Check sheet for the modelled part. Datum: model origin and axes. Units: mm. A direction names the side the tool comes from. Round coordinates to 2 decimals unless told otherwise and drop trailing zeros. Order: outer loops, then holes, each group sorted by start corner. A loop starts at its lowest first (then second) coordinate and runs counter-clockwise, first axis right, second up. Notation, with made-up numbers: (58.5, 9) -> (99.5, 9) arc R24 cw to (99.5, 21) -> close; hole circle Ø1 at (68, 45.5). An arc over 180 degrees is marked (long way). Answer in a Markdown table with one row per item.
Autodesk Fusion 360 part; units mm, degrees
sketch "Sketch1" plane through (0, 0, 0) normal (0, 1, 0) x (1, 0, 0)
  line L0 (17.5, -87.5) -> (-17.5, -87.5)
  line L1 (-17.5, 87.5) -> (17.5, 87.5)
  line L2 (17.5, -87.5) -> (-17.5, 87.5) construction
  line L3 (-17.5, -87.5) -> (17.5, 87.5) construction
  line L4 (-87.5, 17.5) -> (-87.5, -17.5)
  line L5 (87.5, -17.5) -> (87.5, 17.5)
  line L6 (87.5, 17.5) -> (-87.5, -17.5) construction
  line L7 (-87.5, 17.5) -> (87.5, -17.5) construction
  circle A0 centre (-77.5, 12.5) radius 0.5
  circle A1 centre (-77.5, -12.5) radius 0.5
  circle A2 centre (-12.5, -77.5) radius 0.5
  circle A3 centre (12.5, -77.5) radius 0.5
  circle A4 centre (77.5, -12.5) radius 0.5
  circle A5 centre (77.5, 12.5) radius 0.5
  circle A6 centre (-12.5, 77.5) radius 0.5
  circle A7 centre (12.5, 77.5) radius 0.5
  line L8 (-17.5, 87.5) -> (-17.5, 17.5)
  line L9 (17.5, 87.5) -> (17.5, 17.5)
  line L10 (-17.5, -87.5) -> (-17.5, -17.5)
  line L11 (17.5, -87.5) -> (17.5, -17.5)
  line L12 (-87.5, 17.5) -> (-17.5, 17.5)
  line L13 (17.5, 17.5) -> (87.5, 17.5)
  line L14 (87.5, -17.5) -> (17.5, -17.5)
  line L15 (-17.5, -17.5) -> (-87.5, -17.5)
  circle A8 centre (0, 0) radius 0.5
  dimension "d1" = 35
  dimension "d2" = 175
  dimension "d3" = 175
  dimension "d4" = 35
  dimension "d7" = 1
  dimension "d8" = 10
  dimension "d10" = 1
  dimension "d12" = 10
  dimension "d13" = 1
  dimension "d14" = 1
  dimension "d15" = 1
  dimension "d16" = 1
  dimension "d17" = 1
  dimension "d18" = 1
  dimension "d20" = 10
  dimension "d21" = 10
  dimension "d24" = 10
  dimension "d25" = 10
  dimension "d28" = 10
  dimension "d29" = 10
  dimension "d31" = 5
  dimension "d32" = 5
  dimension "d33" = 5
  dimension "d34" = 5
  dimension "d35" = 5
  dimension "d36" = 5
  dimension "d37" = 5
  dimension "d38" = 5
  dimension "d39" = 1
  dimension "d40" = 70
  dimension "d41" = 70
extrude "Extrude1" add sketch "Sketch1" along normal blind 3.93
Item 1: Cross-section at C-C (z = -24). Record the boundary of the cut face in (x, y), and give its area (3 significant figures).
Result sheet:
| item | result |
|---|---|
| outline | (-17.5, 0) -> (17.5, 0) -> (17.5, 3.93) -> (-17.5, 3.93) -> close |
| area | 138 mm^2 |
Item 2: Cross-section at A-A (y = 2). State how many separate pieces and enclosed holes the cut face has, and give its area (3 significant figures).
Result sheet:
| item | result |
|---|---|
| separate pieces | 1 |
| enclosed holes | 9 |
| area | 11,000 mm^2 |
Item 3: Scan lines: line 1 (Z direction, x = 77.5, y = 1.6); line 2 (X direction, y = 1.8, z = -12.5). Record each from-to range of solid material in increasing order. Write a range as [from, to].
Result sheet:
| item | result |
|---|---|
| line 1 | z = [-17.5, -13], [-12, 12], [13, 17.5] |
| line 2 | x = [-87.5, -78], [-77, 77], [78, 87.5] |
Item 4: Set-up check for faces 1 (the flat face through (-53, 2, -17.5)), 2 (the flat face through (-52, 2, 17.5)), 3 (the flat face through (53, 2, 17.5)): record each of +Z, -Z, +X, -X, +Y, -Y from which the full face is reachable in a straight line by a thin tool's end or side.
Result sheet:
| item | result |
|---|---|
| face 1 | -Z, -X, +Y, -Y |
| face 2 | +Z, -X, +Y, -Y |
| face 3 | +Z, +X, +Y, -Y |
Item 5: Depth check by flat-ended pin: P1, Ø1.2, axis at x = -43, y = 1.5, coming from the +Z side; P2, Ø12, axis at x = -19.5, z = 52.5, coming from the +Y side; P3, Ø2, axis at y = 1, z = 69, coming from the +X side; P4, Ø2, axis at y = 2.5, z = -49.5, coming from the -X side. Enter the tip coordinate at first touch or a pass-through.
Result sheet:
| item | result |
|---|---|
| P1 | stops at z = 17.5 |
| P2 | stops at y = 3.93 |
| P3 | stops at x = 17.5 |
| P4 | stops at x = -17.5 |
Item 6: Cross-section at B-B (x = -71.5). Record the boundary of the cut face in (y, z), and give its area (3 significant figures).
Result sheet:
| item | result |
|---|---|
| outline | (0, -17.5) -> (3.93, -17.5) -> (3.93, 17.5) -> (0, 17.5) -> close |
| area | 138 mm^2 |
